Here's the drawing with two shaded views (mm, measured from the low corner). I have some questions. Coordinates: 2 decimals unless noted, no trailing zeros. Loops run counter-clockwise (first coordinate to the right, second up) from the corner with the lowest first, then second, coordinate; pieces in that order, holes last.
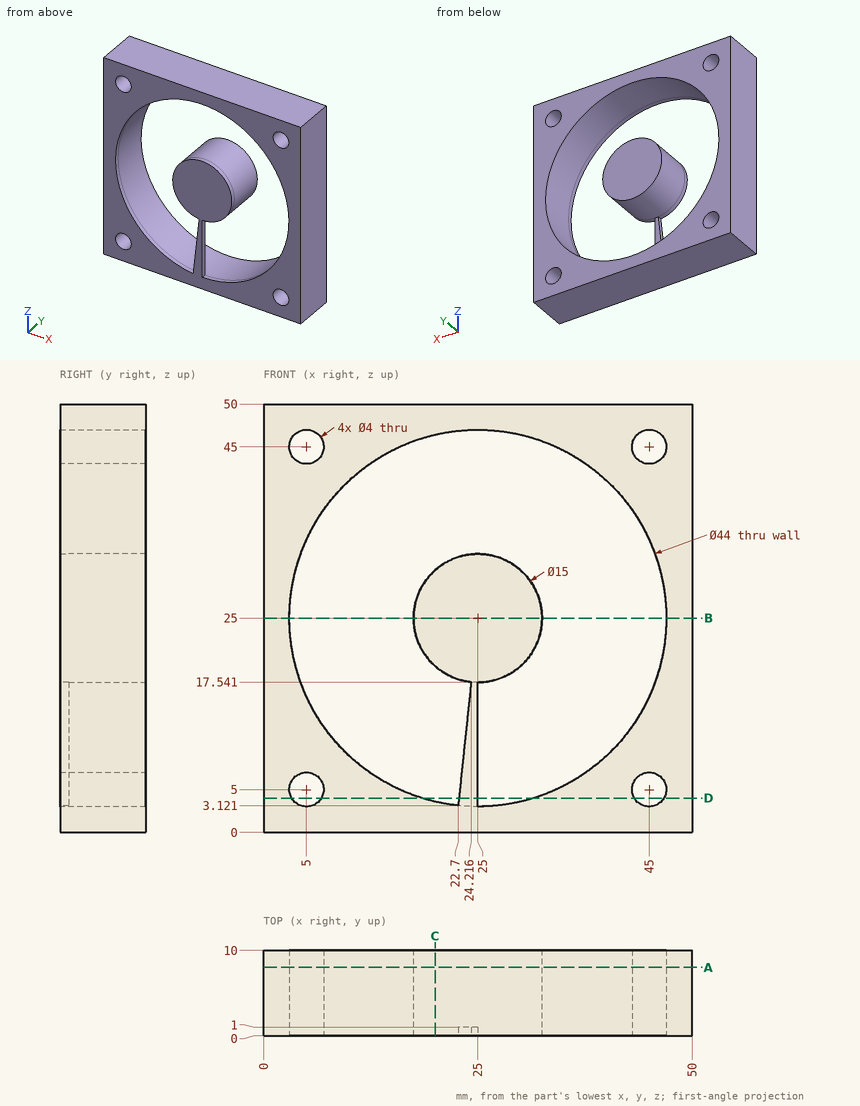
(1) I'm going to push flat-ended pins straight in: pin 1 (3.5 mm diameter, centred on x = 5, z = 45, fed in from +Y); pin 2 (2.5 mm diameter, centred on x = 24.5, z = 9, fed in from +Y). Where does each tip first touch, or does it pass through?
Check values:
pin 1: passes through
pin 2: stops at y = 1
(2) I want a section at B-B on z = 25. Write out the boundary of the cut face in (x, y), then the cut area to 3 significant figures.
Check values:
outline: (0, 0) - (3, 0) - (3, 10) - (0, 10) - close; (17.5, 0) - (32.5, 0) - (32.5, 10) - (17.5, 10) - close; (47, 0) - (50, 0) - (50, 10) - (47, 10) - close
area: 210 mm2
(3) If I drill on probe 1 along X at (y, z) = (0.45, 25); probe 2 along X at (y, z) = (3.5, 5) (1 decimal); probe 3 along X at (y, z) = (1.5, 23), over which ranges is the centre line in solid material (lowest first)?
Check values:
probe 1: x = 0 to 3, 17.5 to 32.5, 47 to 50
probe 2: x = 0 to 3, 7 to 15.8, 34.2 to 43, 47 to 50
probe 3: x = 0 to 3.09, 17.77 to 32.23, 46.91 to 50
(4) I want a section at D-D on z = 4. Write out the boundary of the cut face in (x, y), then the cut area to 3 significant figures.
Check values:
outline: (0, 0) - (3.27, 0) - (3.27, 10) - (0, 10) - close; (6.73, 0) - (18.44, 0) - (18.44, 10) - (6.73, 10) - close; (22.79, 0) - (25, 0) - (25, 1) - (22.79, 1) - close; (31.56, 0) - (43.27, 0) - (43.27, 10) - (31.56, 10) - close; (46.73, 0) - (50, 0) - (50, 10) - (46.73, 10) - close
area: 302 mm2
(5) I want a section at C-C on x = 20. Write out the boundary of the cut face in (y, z) (1 decimal), then the cut area to 3 significant figures.
Check values:
outline: (0, 0) - (10, 0) - (10, 3.6) - (0, 3.6) - close; (0, 19.4) - (10, 19.4) - (10, 30.6) - (0, 30.6) - close; (0, 46.4) - (10, 46.4) - (10, 50) - (0, 50) - close
area: 183 mm2
(6) I want a section at A-A on y = 8. Write out the boundary of the cut face in (x, z).
Check values:
outline: (0, 0) - (50, 0) - (50, 50) - (0, 50) - close; circle Ø15 at (25, 25); hole circle Ø4 at (5, 5); hole circle Ø44 at (25, 25); hole circle Ø4 at (5, 45); hole circle Ø4 at (45, 5); hole circle Ø4 at (45, 45)
